from build123d import *

# Parameters (mm, degrees)
BOSS_EXTRUDE1_DEPTH     = 132.5
SKETCH2_R               = 2.5
CUT_EXTRUDE3_DEPTH      = 132.5
CUT_EXTRUDE3_DEPTH_BACK = 132.5


with BuildPart() as part:
    # Sketch1 → Boss-Extrude1 (new body, symmetric)
    with BuildSketch(Plane.XY):
        Polygon((-2.585786438, 4), (2.585786438, 4), (6.585786438, 8), (2.5, 8), (2.5, 10), (10, 10), (10, 2.5), (8, 2.5), (8, 6.585786438), (4, 2.585786438), (4, -2.585786438), (8, -6.585786438), (8, -2.5), (10, -2.5), (10, -10), (2.5, -10), (2.5, -8), (6.585786438, -8), (2.585786438, -4), (-2.585786438, -4), (-6.585786438, -8), (-2.5, -8), (-2.5, -10), (-10, -10), (-10, -2.5), (-8, -2.5), (-8, -6.585786438), (-4, -2.585786438), (-4, 2.585786438), (-8, 6.585786438), (-8, 2.5), (-10, 2.5), (-10, 10), (-2.5, 10), (-2.5, 8), (-6.585786438, 8), align=None)
    extrude(amount=BOSS_EXTRUDE1_DEPTH, both=True)

    # Sketch2 → Cut-Extrude3 (cut, two sides)
    with BuildSketch(Plane.XY) as cut_extrude3_sk:
        Circle(SKETCH2_R)
    extrude(amount=CUT_EXTRUDE3_DEPTH, mode=Mode.SUBTRACT)
    extrude(cut_extrude3_sk.sketch, amount=-CUT_EXTRUDE3_DEPTH_BACK, mode=Mode.SUBTRACT)


solid = part.part
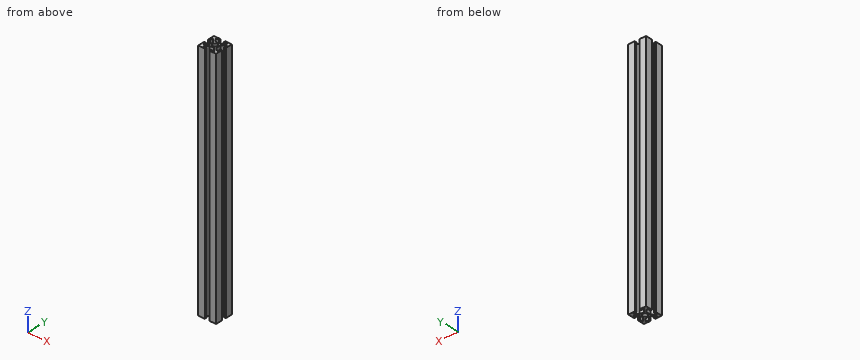
The listing builds one solid part. Answer for the finished solid, in the listing's coordinates (mm). Coordinates: 2 decimals unless noted, no trailing zeros. Loops run counter-clockwise (first coordinate to the right, second up) from the corner with the lowest first, then second, coordinate; pieces in that order, holes last.
1) A flat-ended cylindrical pin translates along its axis: pin 1 Ø1.6 at (y, z) = (-0.5, 63.5) entering from +X. Find the tip coordinate at first contact, or state that the pin passes through.
2) Find the intervals of material crossed by L1, parallel to X at y = 9, z = -69; L2, parallel to Y at x = 0, z = 37.5; L3, parallel to Y at x = 5.25, z = 8.5, in increasing order.
3) Find section A-A on y = 0. Write down the section's boundary in (x, z), then the cut area to 3 significant figures.
Values:
1. pin 1: stops at x = 4
2. L1: x = -10 to -2.5, 2.5 to 10
2. L2: y = -4 to -2.5, 2.5 to 4
2. L3: y = -10 to -8, -6.66 to -3.84, 3.84 to 6.66, 8 to 10
3. outline: (-4, -132.5) - (-2.5, -132.5) - (-2.5, 132.5) - (-4, 132.5) - close; (2.5, -132.5) - (4, -132.5) - (4, 132.5) - (2.5, 132.5) - close
3. area: 795 mm2
